For this review, use the dimensioned drawing (mm, ordinates from the lowest corner) and the shaded views. Coordinates: 2 decimals unless noted, no trailing zeros. Write item = value, one per line. Start each with the question number.
Q1. We need section A-A on z = 8.89. Count the separate pieces of the cut face and the enclosed holes in it, and give its area (3 significant figures).
Q2. Wall thickness on probe 1 along X at (y, z) = (20.5, 5.25) (1 decimal); probe 2 along Y at (x, z) = (98.5, 13.5); probe 3 along X at (y, z) = (8, 3.75): over which ranges is each line inside the solid? List them lowest first.
Q3. Clearance check with flat-ended pins moving along their axes: pin 1 Ø7 at (y, z) = (2.5, 11.5) entering from +X; pin 2 Ø10 at (y, z) = (26.5, 14) entering from +X; pin 3 Ø2 at (y, z) = (23, 12) entering from +X (1 decimal). State where each tip first meets the part, or that it passes through.
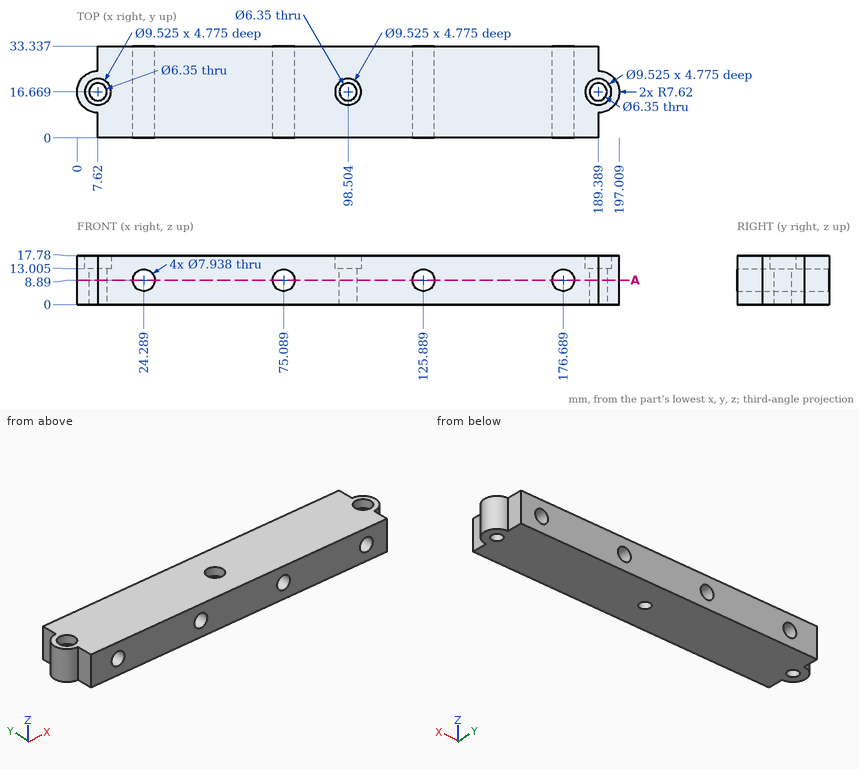
Returned:
q1.separate_pieces = 5
q1.enclosed_holes = 3
q1.area = 5,090 mm^2
q2.probe_1 = 1 to 22.7, 25.9 to 73.5, 76.7 to 124.3, 127.5 to 175.1, 178.3 to 196
q2.probe_2 = 0 to 11.91, 21.43 to 33.34
q2.probe_3 = 7.62 to 189.39
q3.pin_1 = 189.39
q3.pin_2 = 195.28
q3.pin_3 = 194.8
